from build123d import *
from build123d.topology import SkipClean

# Parameters (mm, degrees)
CROQUIS1_R              = 75
SALIENTE_EXTRUIR1_DEPTH = 15
SALIENTE_EXTRUIR2_START = 50
SALIENTE_EXTRUIR2_DEPTH = 50
CROQUIS3_R              = 75
CROQUIS3_R_2            = 60
SALIENTE_EXTRUIR3_DEPTH = 20
CROQUIS4_R              = 25
CORTAR_EXTRUIR1_DEPTH   = 20


with BuildPart() as part:
    # Croquis1 → Saliente-Extruir1 (new body)
    with BuildSketch(Plane.XY):
        Circle(CROQUIS1_R)
    extrude(amount=SALIENTE_EXTRUIR1_DEPTH)

    # Croquis2 → Saliente-Extruir2 (add)
    with SkipClean():  # the faces are left unmerged after this step: merging them gives an invalid solid
        with BuildSketch(Plane(origin=(0, 0, 0), x_dir=(-1, 0, 0), z_dir=(0, 0, -1)).offset(SALIENTE_EXTRUIR2_START)):
            with BuildLine():
                Line((-70.710678119, 25), (0, 25))
                Line((0, 25), (0, 40))
                Line((0, 40), (-63.442887702, 40))
                ThreePointArc((-63.442887702, 40), (-67.494776136, 32.70252581), (-70.710678119, 25))
            make_face()
            with BuildLine():
                Line((0, 40), (0, 25))
                Line((0, 25), (70.710678119, 25))
                ThreePointArc((70.710678119, 25), (67.494776136, 32.70252581), (63.442887702, 40))
                Line((63.442887702, 40), (0, 40))
            make_face()
            with BuildLine():
                Line((-70.710678119, 25), (0, 25))
                Line((0, 25), (0, 40))
                Line((0, 40), (-63.442887702, 40))
                ThreePointArc((-63.442887702, 40), (-67.494776136, 32.70252581), (-70.710678119, 25))
            make_face()
            with BuildLine():
                Line((0, -40), (0, -25))
                Line((0, -25), (-70.710678119, -25))
                ThreePointArc((-70.710678119, -25), (-67.494776136, -32.70252581), (-63.442887702, -40))
                Line((-63.442887702, -40), (0, -40))
            make_face()
            with BuildLine():
                Line((70.710678119, -25), (0, -25))
                Line((0, -25), (0, -40))
                Line((0, -40), (63.442887702, -40))
                ThreePointArc((63.442887702, -40), (67.494776136, -32.70252581), (70.710678119, -25))
            make_face()
            with BuildLine():
                Line((0, -40), (0, -25))
                Line((0, -25), (-70.710678119, -25))
                ThreePointArc((-70.710678119, -25), (-67.494776136, -32.70252581), (-63.442887702, -40))
                Line((-63.442887702, -40), (0, -40))
            make_face()
            with BuildLine():
                Line((70.710678119, -25), (0, -25))
                Line((0, -25), (0, -40))
                Line((0, -40), (63.442887702, -40))
                ThreePointArc((63.442887702, -40), (67.494776136, -32.70252581), (70.710678119, -25))
            make_face()
        extrude(amount=-SALIENTE_EXTRUIR2_DEPTH)

    # Croquis3 → Saliente-Extruir3 (add)
    with SkipClean():  # the faces are left unmerged after this step: merging them gives an invalid solid
        with BuildSketch(Plane.XY.offset(15)):
            with Locations(Location((0, 0, 0), (0, 0, 160.528779366))):
                Circle(CROQUIS3_R)
            Circle(CROQUIS3_R_2, mode=Mode.SUBTRACT)
        extrude(amount=SALIENTE_EXTRUIR3_DEPTH)

    # Croquis4 → Cortar-Extruir1 (cut)
    with SkipClean():  # the faces are left unmerged after this step: merging them gives an invalid solid
        with BuildSketch(Plane.XY.offset(15)):
            Circle(CROQUIS4_R)
        extrude(amount=-CORTAR_EXTRUIR1_DEPTH, mode=Mode.SUBTRACT)


solid = part.part
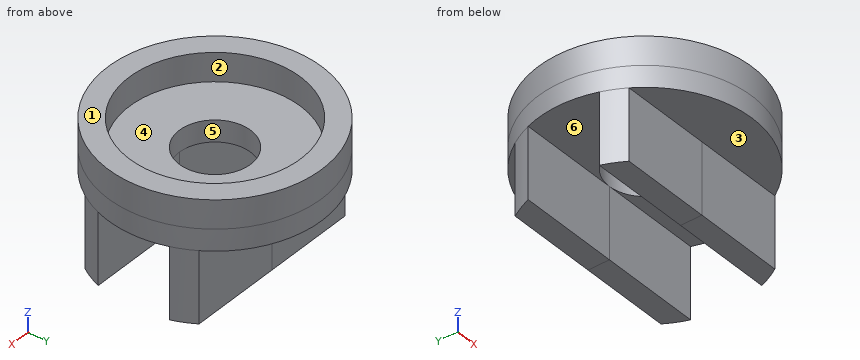
Can you work these out from the model? Positions are in its coordinate system, mm. Face numbers are marked on the shaded views. A direction names the side the tool comes from. Round coordinates to 2 decimals unless told otherwise and drop trailing zeros. Write each loop counter-clockwise with the first axis right and the second up, starting at its lowest first coordinate (ties: lowest second). Pieces come first, ordered by that corner, then holes. Notation, with made-up numbers: (0.5, 63) -> (55.5, 63) arc R20 cw to (55.5, 100) -> close; hole circle Ø11 at (52.5, 5). An arc over 180 degrees is marked (long way). One line per question, with ' | ' between items. Start each with the question number.
1) Suppose I cut it at A-A on y = 0. Write out the boundary of the cut face in (x, z).
2) On a 3-axis mill with a long thin cutter (end or side, diameter ignored), from which of +Z, -Z, +X, -X, +Y, -Y can I reach the whole of each face in a straight line? I mean the marked faces 1, 2 and 3. Say none if no direction works.
3) I'm going to push flat-ended pins straight in: P1, Ø4, axis at y = 19.5, z = 25.5, coming from the +X side; P2, Ø5, axis at x = -49.5, z = 13, coming from the +Y side; P3, Ø1.5, axis at y = 36, z = 6, coming from the -X side. Where does each tip first touch, or does it pass through?
4) Suppose I cut it at B-B on z = -10.5. Write out the boundary of the cut face in (x, y), then the cut area to 3 significant figures.
5) If we mould it in two halves opening along X, with no side actions, what happens to the marked faces 4, 5 and 6? For each: released by +X, released by -X, zero draft, split by the parting line, or undercut.
6) Suppose I cut it at D-D on y = -53. Write out the boundary of the cut face in (x, z), then the cut area to 3 significant figures.
7) I need wall thicknesses on line 1 (Y direction, x = 6.5, z = -30); line 2 (Y direction, x = 0, z = 25); line 3 (Z direction, x = -36, y = 50). Which ranges of each line are inside material? Lowest first, please. Write a range as [from, to].
8) Suppose I cut it at C-C on x = -8. Write out the boundary of the cut face in (y, z), then the cut area to 3 significant figures.
Return value:
1) outline: (-75, 0) -> (-25, 0) -> (-25, 15) -> (-60, 15) -> (-60, 35) -> (-75, 35) -> close; (25, 0) -> (75, 0) -> (75, 35) -> (60, 35) -> (60, 15) -> (25, 15) -> close
2) face 1: +Z, +X, -X, +Y, -Y | face 2: +Z | face 3: -Z, +X, -X, -Y
3) P1: stops at x = 72.93 | P2: stops at y = 58.45 | P3: stops at x = -66.2
4) outline: (-70.71, -25) arc R75 ccw to (-63.44, -40) -> (63.44, -40) arc R75 ccw to (70.71, -25) -> close; (-70.71, 25) -> (70.71, 25) arc R75 ccw to (63.44, 40) -> (-63.44, 40) arc R75 ccw to start | area: 4,050 mm2
5) face 4: undercut | face 5: undercut | face 6: zero draft
6) outline: (-53.07, 0) -> (53.07, 0) -> (53.07, 35) -> (28.12, 35) -> (28.12, 15) -> (-28.12, 15) -> (-28.12, 35) -> (-53.07, 35) -> close | area: 2,590 mm2
7) line 1: y = [-40, -25], [25, 40] | line 2: y = [-75, -60], [60, 75] | line 3: z = [0, 35]
8) outline: (-74.57, 0) -> (-40, 0) -> (-40, -50) -> (-25, -50) -> (-25, 0) -> (-23.69, 0) -> (-23.69, 15) -> (-59.46, 15) -> (-59.46, 35) -> (-74.57, 35) -> close; (23.69, 0) -> (25, 0) -> (25, -50) -> (40, -50) -> (40, 0) -> (74.57, 0) -> (74.57, 35) -> (59.46, 35) -> (59.46, 15) -> (23.69, 15) -> close | area: 3,630 mm2
